Work out the finished part from the listing and answer in its coordinate system (mm). A direction names the side the tool comes from. Give positions to 0.01 mm unless a question says otherwise; leave off trailing zeros. Loops run counter-clockwise (first coordinate to the right, second up) from the corner with the lowest first, then second, coordinate; pieces in that order, holes last. Notation, with made-up numbers: (9, 32.5) - (62, 32.5) arc R21 cw to (62, 62.5) - close; hole circle Ø3 at (-20, 11.25). An arc over 180 degrees is marked (long way). One line per question, with ' | ' between items. Start each with the question number.
1. For a pull along Z with two mould halves and no side action, classify faces 5 (the face through (26, 6, -62)), 6 (the face through (22.5, 8, -63)), 7 (the face through (12, 3, -26)), 8 (the face through (4, 7, -51)) as released by +Z, released by -Z, zero draft, split by the parting line, or undercut.
2. Section A-A (z = -90) is taken. Determine the outline of the cut face in (x, y), plus the area to 3 significant figures.
3. Each of these flat-tipped pins is pushed along its axis until it touches: pin 1 (0.8 mm diameter, centred on x = 11, y = 5.5, fed in from +Z); pin 2 (5 mm diameter, centred on x = 5, y = 41, fed in from +Z); pin 3 (2.5 mm diameter, centred on y = 7.5, z = -48, fed in from -X). Where does it stop, or does it pass through?
4. Find the intervals of material crossed by line 1 (X direction, y = 49.25, z = -56); line 2 (X direction, y = 3.6, z = -22); line 3 (X direction, y = 45.5, z = -55), in increasing order.
5. Section C-C (y = 43) is taken. Determine the outline of the cut face in (x, z).
6. Section D-D (z = -56) is taken. Determine the outline of the cut face in (x, y), plus the area to 3 significant figures.
7. Section B-B (x = 15) is taken. Determine the outline of the cut face in (y, z), plus the area to 3 significant figures.
8. Which of the six approach directions +Z, -Z, +X, -X, +Y, -Y give full straight-line access (tool end or side, diameter ignored) to faces 1 (the face through (12.5, 8, -49)), 2 (the face through (15, 6, -62)), 3 (the face through (22.5, 8, -49)), 4 (the face through (7.5, 8, -63))?
from build123d import *

# Parameters (mm, degrees)
SKETCH1_W                = 60
SKETCH1_H                = 5
BOSS_EXTRUDE1_DEPTH      = 30
SKETCH2_W                = 30
SKETCH2_H                = 8
BOSS_EXTRUDE2_DEPTH      = 47
SKETCH3_R                = 5
CUT_EXTRUDE1_DEPTH       = 82.908485519
SKETCH5_R                = 1.6
CUT_EXTRUDE3_DEPTH       = 14
FILLET1_R                = 5
FILLET2_R                = 5
SKETCH6_W                = 5
SKETCH6_H                = 5
SKETCH6_H_2              = 3
SKETCH6_H_3              = 8
BOSS_EXTRUDE3_DEPTH      = 9
CHAMFER1_SIZE            = 8
CHAMFER1_OF_MIRROR2_SIZE = 8


with BuildPart() as part:
    # Sketch1 → Boss-Extrude1 (new body)
    with BuildSketch(Plane(origin=(0, 0, 0), x_dir=(0, 0, -1), z_dir=(1, 0, 0))):
        with Locations((30, 2.5)):
            Rectangle(SKETCH1_W, SKETCH1_H)
    boss_extrude1 = extrude(amount=BOSS_EXTRUDE1_DEPTH)

    # Sketch2 → Boss-Extrude2 (add)
    with BuildSketch(Plane(origin=(0, 5, 0), x_dir=(1, 0, 0), z_dir=(0, 1, 0))):
        with Locations((15, 56)):
            Rectangle(SKETCH2_W, SKETCH2_H)
    extrude(amount=BOSS_EXTRUDE2_DEPTH)

    # Sketch3 → Cut-Extrude1 (cut, through all)
    with BuildSketch(Plane(origin=(0, 5, 0), x_dir=(1, 0, 0), z_dir=(0, 1, 0))):
        with Locations(Location((15, 22, 0), (0, 0, 270))):
            Circle(SKETCH3_R)
    cut_extrude1 = extrude(amount=-CUT_EXTRUDE1_DEPTH, mode=Mode.SUBTRACT)

    # Sketch5 → Cut-Extrude3 (cut)
    with BuildSketch(Plane(origin=(0, 52, 0), x_dir=(1, 0, 0), z_dir=(0, 1, 0))):
        with Locations(Location((5, 56, 0), (0, 0, 270))):
            Circle(SKETCH5_R)
        with Locations(Location((25, 56, 0), (0, 0, 270))):
            Circle(SKETCH5_R)
    extrude(amount=-CUT_EXTRUDE3_DEPTH, mode=Mode.SUBTRACT)

    # Fillet1
    fillet1_edges = [part.edges().sort_by_distance(p)[0] for p in [
        (15, 5, -52),
        (30, 2.5, 0),
        (0, 2.5, 0),
        (15, 0, -60),
    ]]
    fillet(fillet1_edges, radius=FILLET1_R)

    # Mirror1: Boss-Extrude1, Cut-Extrude1 across plane
    add(boss_extrude1.mirror(Plane(origin=(0, 0, -56), x_dir=(1, 0, 0), z_dir=(0, 0, -1))))
    add(cut_extrude1.mirror(Plane(origin=(0, 0, -56), x_dir=(1, 0, 0), z_dir=(0, 0, -1))), mode=Mode.SUBTRACT)

    # Fillet2
    fillet2_edges = [part.edges().sort_by_distance(p)[0] for p in [
        (15, 5, -60),
        (0, 2.5, -112),
        (30, 2.5, -112),
    ]]
    fillet(fillet2_edges, radius=FILLET2_R)

    # Sketch6 → Boss-Extrude3 (add)
    with BuildSketch(Plane(origin=(0, 5, 0), x_dir=(1, 0, 0), z_dir=(0, 1, 0))):
        with Locations((20, 49.5)):
            Rectangle(SKETCH6_W, SKETCH6_H)
        with Locations((20, 45.5)):
            Rectangle(SKETCH6_W, SKETCH6_H_2)
        with Locations((10, 48)):
            Rectangle(SKETCH6_W, SKETCH6_H_3)
    boss_extrude3 = extrude(amount=BOSS_EXTRUDE3_DEPTH)

    # Chamfer1
    chamfer1_edges = [part.edges().sort_by_distance(p)[0] for p in [
        (20, 14, -44),
        (10, 14, -44),
    ]]
    chamfer(chamfer1_edges, length=CHAMFER1_SIZE - 0.0001)  # a hair under: the kernel refuses the full size

    # Mirror2: Boss-Extrude3 across plane
    add(boss_extrude3.mirror(Plane(origin=(0, 0, -56), x_dir=(1, 0, 0), z_dir=(0, 0, -1))))

    # Chamfer1 of Mirror2
    chamfer1_of_mirror2_edges = [part.edges().sort_by_distance(p)[0] for p in [
        (20, 14, -68),
        (10, 14, -68),
    ]]
    chamfer(chamfer1_of_mirror2_edges, length=CHAMFER1_OF_MIRROR2_SIZE - 0.0001)  # a hair under: the kernel refuses the full size


solid = part.part
Conclusion:
1) face 5: released by -Z | face 6: zero draft | face 7: undercut | face 8: released by +Z
2) outline: (0, 0) - (10, 0) - (10, 5) - (0, 5) - close; (20, 0) - (30, 0) - (30, 5) - (20, 5) - close | area: 100 mm²
3) pin 1: z = -44 | pin 2: z = -52 | pin 3: x = 7.5
4) line 1: 0 to 3.4, 6.6 to 23.4, 26.6 to 30 | line 2: 0 to 10, 20 to 30 | line 3: 0 to 3.75, 6.25 to 23.75, 26.25 to 30
5) outline: (0, -60) - (30, -60) - (30, -52) - (0, -52) - close; hole circle Ø3.2 at (5, -56); hole circle Ø3.2 at (25, -56)
6) outline: (0, 0) - (30, 0) - (30, 52) - (26.6, 52) - (26.6, 38) - (23.4, 38) - (23.4, 52) - (6.6, 52) - (6.6, 38) - (3.4, 38) - (3.4, 52) - (0, 52) - close | area: 1,470 mm²
7) outline: (0, -112) - (5, -112) - (5, -95) - (0, -95) - close; (0, -85) - (5, -85) - (5, -65) arc R5 cw to (10, -60) - (52, -60) - (52, -52) - (10, -52) arc R5 cw to (5, -47) - (5, -27) - (0, -27) - close; (0, -17) - (5, -17) - (5, 0) - (0, 0) - close | area: 847 mm²
8) face 1: +Z, +Y | face 2: -Z, +Y | face 3: +Z, +X, +Y | face 4: -Z, -X, +Y
